Part model, mm, in its own coordinate system. Face numbers are marked on the shaded views. A direction names the side the tool comes from. Round coordinates to 2 decimals unless told otherwise and drop trailing zeros. Loops run counter-clockwise (first coordinate to the right, second up) from the corner with the lowest first, then second, coordinate; pieces in that order, holes last.
(1) Cut at C-C on y = 83.5. List the corners of the cut face in (x, z) (3 decimals).
(2) Mould opens along Z. For the marked faces 1, 2 and 3 say: +Z half, -Z half, draft (parallel to the pull), parting line (faces both ways), or undercut.
(3) Flat gauge pins, fed straight in: pin 1 (1.8 mm diameter, centred on y = 3, z = 1, fed in from -X); pin 2 (15 mm diameter, centred on y = -101.5, z = 19.5, fed in from +X) (3 decimals); pin 3 (6 mm diameter, centred on x = -27, y = 67.5, fed in from +Z). Where does each tip first touch, or does it go through?
(4) Cut at D-D on x = -65. List the corners of the cut face in (y, z).
(5) Cut at B-B on z = 9.5. List the corners of the cut face in (x, y) (1 decimal).
(6) Cut at A-A on y = -9. List the corners of the cut face in (x, z).
(7) Tool access for the marked faces 4 and 5: list every direction of +Z, -Z, +X, -X, +Y, -Y with a clear straight run to the whole face (end or side of a thin tool).
(8) Probe probe 1 along Y at (x, z) = (-57.15, 0.65); probe 2 along Z at (x, y) = (-46.5, 27.5); probe 3 along X at (y, z) = (86, 35) (3 decimals). List the from-to ranges inside material, lowest first.
from build123d import *

# Parameters (mm, degrees)
BASE_FLANGE1_DEPTH                    = 2.3114
EDGE_FLANGE2_DEPTH                    = 38.1
EDGE_FLANGE3_START                    = -112.7125
EDGE_FLANGE3_DEPTH                    = 38.1
EDGE_FLANGE3_2_DEPTH                  = 38.1
CUT_EXTRUDE1_DEPTH                    = 149.767894723
CUT_EXTRUDE1_DEPTH_BACK               = 149.767894723
BREAK_CORNER1_START                   = -89.191903794
BREAK_CORNER1_DEPTH                   = 2.3114
BREAK_CORNER2_DEPTH                   = 2.3114
F_30_0_1285_DIAMETER_HOLE1_AT_2_COUNT = 2
F_30_0_1285_DIAMETER_HOLE1_AT_2_PITCH = 127
F_30_0_1285_DIAMETER_HOLE1_AT_3_COUNT = 2
F_30_0_1285_DIAMETER_HOLE1_AT_3_PITCH = 119.811560377


# Read off the part's stored shape, not the designer's step: Edge-Flange3, Break-Corner1, Break-Corner2
# Sheet-metal steps are written as plain solids
with BuildPart() as part:
    # Sketch1 → Base-Flange1 (new body)
    with BuildSketch(Plane.XY):
        Polygon((-82.55, 112.7125), (-82.55, -112.7125), (-44.45, -112.7125), (82.55, -20.6375), (82.55, 20.6375), (-44.45, 112.7125), align=None)
    extrude(amount=BASE_FLANGE1_DEPTH)

    # Edge-Flange2 section (across the edge) → Edge-Flange2 (add)
    with BuildSketch(Plane(origin=(-85.725, -74.6125, 2.3114), x_dir=(1, 0, 0), z_dir=(0, -1, 0))):
        with BuildLine():
            Line((-2.3114, 3.175), (-2.3114, 38.1))
            Line((-2.3114, 38.1), (0, 38.1))
            Line((0, 38.1), (0, 3.175))
            ThreePointArc((0, 3.175), (0.92993597, 0.92993597), (3.175, 0))
            Line((3.175, 0), (3.175, -2.3114))
            ThreePointArc((3.175, -2.3114), (-0.704470644, -0.704470644), (-2.3114, 3.175))
        make_face()
    edge_flange2 = extrude(amount=EDGE_FLANGE2_DEPTH)

    # Mirror1: Edge-Flange2 across plane
    add(edge_flange2.mirror(Plane.ZX))

    # Edge-Flange3 outline → Edge-Flange3 (cut)
    with BuildSketch(Plane(origin=(0, 0, 0), x_dir=(1, 0, 0), z_dir=(0, 1, 0)).offset(EDGE_FLANGE3_START)):
        with BuildLine():
            Line((-85.725, -40.4114), (-86.429470644, -39.706929356))
            ThreePointArc((-86.429470644, -39.706929356), (-87.618772667, -37.927013095), (-88.0364, -35.827458711))
            Line((-88.0364, -35.827458711), (-88.0364, -40.4114))
            Line((-88.0364, -40.4114), (-85.725, -40.4114))
        make_face()
    edge_flange3 = extrude(amount=EDGE_FLANGE3_DEPTH, mode=Mode.SUBTRACT)

    # Edge-Flange3 2 outline → Edge-Flange3 2 (add)
    with BuildSketch(Plane(origin=(0, 0, 0), x_dir=(1, 0, 0), z_dir=(0, 1, 0)).offset(EDGE_FLANGE3_START)):
        with BuildLine():
            Line((-85.725, -35.827458711), (-85.725, -40.4114))
            Line((-85.725, -40.4114), (-82.869278554, -43.267121446))
            Line((-82.869278554, -43.267121446), (-81.234871939, -41.632714832))
            Line((-81.234871939, -41.632714832), (-84.79506403, -38.072522742))
            ThreePointArc((-84.79506403, -38.072522742), (-85.483317516, -37.042478609), (-85.725, -35.827458711))
        make_face()
    edge_flange3_2 = extrude(amount=EDGE_FLANGE3_2_DEPTH)

    # Mirror2: Edge-Flange3, Edge-Flange3 2 across plane
    add(edge_flange3.mirror(Plane.ZX), mode=Mode.SUBTRACT)
    add(edge_flange3_2.mirror(Plane.ZX))

    # Sketch15 → Cut-Extrude1 (cut, two sides: drawn at the far end of the back side and taken through both)
    with BuildSketch(Plane.XY.offset(2.3114).offset(-CUT_EXTRUDE1_DEPTH_BACK)):
        with BuildLine():
            Line((71.4375, 12.7), (71.4375, -12.7))
            ThreePointArc((71.4375, -12.7), (69.85, -14.2875), (68.2625, -12.7))
            Line((68.2625, -12.7), (68.2625, 12.7))
            ThreePointArc((68.2625, 12.7), (69.85, 14.2875), (71.4375, 12.7))
        make_face()
    extrude(amount=CUT_EXTRUDE1_DEPTH + CUT_EXTRUDE1_DEPTH_BACK, mode=Mode.SUBTRACT)

    # Break-Corner1 outline → Break-Corner1 (cut)
    with BuildSketch(Plane(origin=(0, 0, 0), x_dir=(0.707106781186541, 0, 0.707106781186554), z_dir=(0.707106781186554, 0, -0.707106781186541)).offset(BREAK_CORNER1_START)):
        with BuildLine():
            Line((-28.00295384, 74.6125), (-28.00295384, 77.7875))
            ThreePointArc((-28.00295384, 77.7875), (-28.93288981, 75.54243597), (-31.17795384, 74.6125))
            Line((-31.17795384, 74.6125), (-28.00295384, 74.6125))
        make_face()
        with BuildLine():
            ThreePointArc((-31.17795384, 112.7125), (-28.93288981, 111.78256403), (-28.00295384, 109.5375))
            Line((-28.00295384, 109.5375), (-28.00295384, 112.7125))
            Line((-28.00295384, 112.7125), (-31.17795384, 112.7125))
        make_face()
        with BuildLine():
            ThreePointArc((-31.17795384, -74.6125), (-28.93288981, -75.54243597), (-28.00295384, -77.7875))
            Line((-28.00295384, -77.7875), (-28.00295384, -74.6125))
            Line((-28.00295384, -74.6125), (-31.17795384, -74.6125))
        make_face()
        with BuildLine():
            ThreePointArc((-28.00295384, -109.5375), (-28.93288981, -111.78256403), (-31.17795384, -112.7125))
            Line((-31.17795384, -112.7125), (-28.00295384, -112.7125))
            Line((-28.00295384, -112.7125), (-28.00295384, -109.5375))
        make_face()
    extrude(amount=BREAK_CORNER1_DEPTH, mode=Mode.SUBTRACT)

    # Break-Corner2 outline → Break-Corner2 (cut)
    with BuildSketch(Plane.XY):
        with BuildLine():
            Line((-44.45, 112.7125), (-48.569388338, 112.7125))
            ThreePointArc((-48.569388338, 112.7125), (-44.650974655, 112.09289876), (-41.114900181, 110.294552631))
            Line((-41.114900181, 110.294552631), (-44.45, 112.7125))
        make_face()
        with BuildLine():
            Line((-44.45, -112.7125), (-41.114900181, -110.294552631))
            ThreePointArc((-41.114900181, -110.294552631), (-44.650974655, -112.09289876), (-48.569388338, -112.7125))
            Line((-48.569388338, -112.7125), (-44.45, -112.7125))
        make_face()
        with BuildLine():
            Line((82.55, -20.6375), (82.55, -14.158443455))
            ThreePointArc((82.55, -14.158443455), (81.16286877, -19.929838451), (77.304488158, -24.440496086))
            Line((77.304488158, -24.440496086), (82.55, -20.6375))
        make_face()
        with BuildLine():
            Line((82.55, 20.6375), (77.304488158, 24.440496086))
            ThreePointArc((77.304488158, 24.440496086), (81.16286877, 19.929838451), (82.55, 14.158443455))
            Line((82.55, 14.158443455), (82.55, 20.6375))
        make_face()
    extrude(amount=BREAK_CORNER2_DEPTH, mode=Mode.SUBTRACT)

    # Sketch18 → #30 (0.1285) Diameter Hole1 (revolve, cut)
    with BuildSketch(Plane(origin=(-57.15, -63.5, 2.3114), x_dir=(0, -1, 0), z_dir=(1, 0, 0))):
        Polygon((0, 0), (0, 2.3114), (1.63195, 2.3114), (1.63195, 1.54132111), (2.9718, 0), align=None)
    f_30_0_1285_diameter_hole1 = revolve(axis=Axis((-57.15, -63.5, 8.6614), (0, 0, -1)), mode=Mode.SUBTRACT)

    # #30 (0.1285) Diameter Hole1 at 2: #30 (0.1285) Diameter Hole1 ×2
    with Locations(*[(0, i * F_30_0_1285_DIAMETER_HOLE1_AT_2_PITCH, 0) for i in range(1, F_30_0_1285_DIAMETER_HOLE1_AT_2_COUNT)]):
        add(f_30_0_1285_diameter_hole1, mode=Mode.SUBTRACT)

    # #30 (0.1285) Diameter Hole1 at 3: #30 (0.1285) Diameter Hole1 ×2
    with Locations(*[Vector(0.8479983040050879, 0.52999894000318, 0) * (i * F_30_0_1285_DIAMETER_HOLE1_AT_3_PITCH) for i in range(1, F_30_0_1285_DIAMETER_HOLE1_AT_3_COUNT)]):
        add(f_30_0_1285_diameter_hole1, mode=Mode.SUBTRACT)


solid = part.part
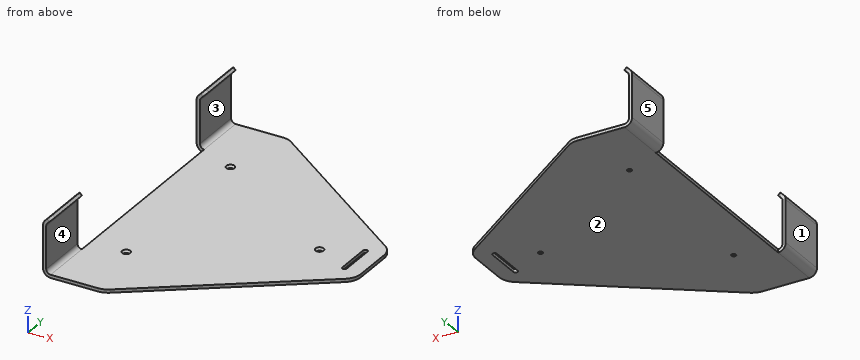
Final values:
1. outline: (-88.036, 5.486) arc R5.486 ccw to (-82.55, 0) - (-4.157, 0) - (-4.157, 2.311) - (-82.55, 2.311) arc R3.175 cw to (-85.725, 5.486) - (-85.725, 35.827) arc R3.175 cw to (-84.795, 38.073) - (-81.235, 41.633) - (-82.869, 43.267) - (-86.429, 39.707) arc R5.486 ccw to (-88.036, 35.827) - close
2. face 1: draft
2. face 2: -Z half
2. face 3: undercut
3. pin 1: stops at x = -82.55
3. pin 2: stops at x = -85.725
3. pin 3: stops at z = 2.31
4. outline: (-112.71, 0) - (112.71, 0) - (112.71, 2.31) - (-112.71, 2.31) - close
5. outline: (-88, -112.7) - (-85.7, -112.7) - (-85.7, -74.6) - (-88, -74.6) - close; (-88, 74.6) - (-85.7, 74.6) - (-85.7, 112.7) - (-88, 112.7) - close
6. outline: (-82.55, 0) - (68.26, 0) - (68.26, 2.31) - (-82.55, 2.31) - close; (71.44, 0) - (82.55, 0) - (82.55, 2.31) - (71.44, 2.31) - close
7. face 4: +X, +Y, -Y
7. face 5: +Z, -Z, -X, +Y, -Y
8. probe 1: y = -112.71 to -65.13, -61.87 to 61.87, 65.13 to 112.71
8. probe 2: z = 0 to 2.31
8. probe 3: x = -88.036 to -85.725
